The figure shows three views and two pictorial views of one solid part (mm, origin at its lowest corner). Answer the questions. Coordinates: 2 decimals unless noted, no trailing zeros. Loops run counter-clockwise (first coordinate to the right, second up) from the corner with the lowest first, then second, coordinate; pieces in that order, holes last. Notation, with made-up numbers: (20.25, 67.25) - (60.25, 67.25) arc R21 cw to (60.25, 77.25) - close; hole circle Ø1 at (-27.5, 12.5). An arc over 180 degrees is marked (long way). One line per question, with ' | ' between items.
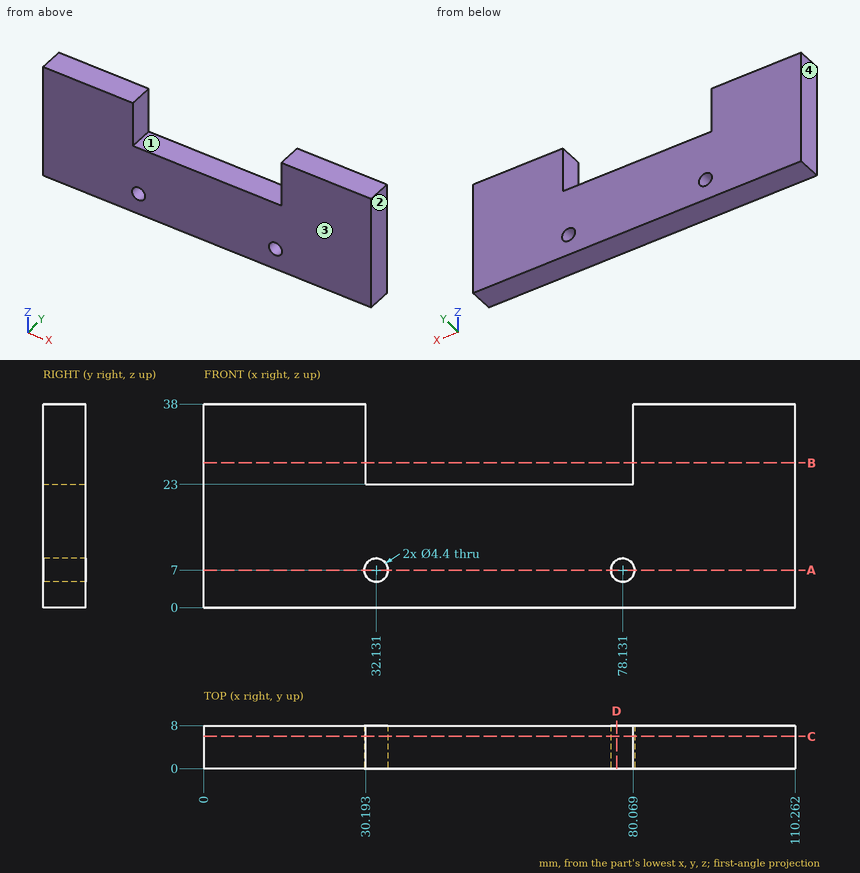
Item 1: The mould has two halves that part along X. Classify the marked faces 1, 2, 3 and 4: pulls with the +X half, pulls with the -X half, needs draft (parallel to the pull), parting line crosses it, or undercut.
Taken from the geometry:
face 1: undercut | face 2: pulls with the +X half | face 3: needs draft | face 4: pulls with the -X half
Item 2: Find section D-D, the plane x = 77. Write down the section's boundary in (y, z).
Taken from the geometry:
outline: (0, 0) - (8, 0) - (8, 5.11) - (0, 5.11) - close; (0, 8.89) - (8, 8.89) - (8, 23) - (0, 23) - close
Item 3: Find the intervals of material crossed by line 1 (X direction, y = 3.5, z = 7); line 2 (X direction, y = 1.5, z = 8.5); line 3 (X direction, y = 6.75, z = 32), in increasing order. Write a range as [from, to].
Taken from the geometry:
line 1: x = [0, 29.93], [34.33, 75.93], [80.33, 110.26] | line 2: x = [0, 30.52], [33.74, 76.52], [79.74, 110.26] | line 3: x = [0, 30.19], [80.07, 110.26]
Item 4: Find section B-B, the plane z = 27. Write down the section's boundary in (x, y).
Taken from the geometry:
outline: (0, 0) - (30.19, 0) - (30.19, 8) - (0, 8) - close; (80.07, 0) - (110.26, 0) - (110.26, 8) - (80.07, 8) - close
Item 5: Find section C-C, the plane y = 6. Write down the section's boundary in (x, z).
Taken from the geometry:
outline: (0, 0) - (110.26, 0) - (110.26, 38) - (80.07, 38) - (80.07, 23) - (30.19, 23) - (30.19, 38) - (0, 38) - close; hole circle Ø4.4 at (32.13, 7); hole circle Ø4.4 at (78.13, 7)
Item 6: Each of these flat-tipped pins is pushed along its axis until it touches: pin 1 Ø4 at (x, y) = (61, 3) entering from +Z; pin 2 Ø2.5 at (x, z) = (32.13, 7) entering from -Y. Where does it stop, or does it pass through?
Taken from the geometry:
pin 1: stops at z = 23 | pin 2: passes through
Item 7: Find section A-A, the plane z = 7. Write down the section's boundary in (x, y).
Taken from the geometry:
outline: (0, 0) - (29.93, 0) - (29.93, 8) - (0, 8) - close; (34.33, 0) - (75.93, 0) - (75.93, 8) - (34.33, 8) - close; (80.33, 0) - (110.26, 0) - (110.26, 8) - (80.33, 8) - close
